Drawing for the job (mm, zero at the part's lowest x, y, z). A direction names the side the tool comes from. Round coordinates to 2 decimals unless told otherwise and drop trailing zeros. Order: outer loops, then holes, each group sorted by start corner. A loop starts at its lowest first (then second) coordinate and runs counter-clockwise, first axis right, second up. Notation, with made-up numbers: (85, 33) - (130, 33) arc R13 ccw to (130, 56) - close; hole circle Ø11 at (59, 50). An arc over 180 degrees is marked (long way). Put each result on its own line as item: value. Start each with the question number.
Item 1: Saw through at D-D on z = 3.65. List the corners of the cut face in (x, y), plus the area to 3 significant figures.
Item 2: Saw through at A-A on z = 2.25. List the corners of the cut face in (x, y), plus the area to 3 significant figures.
Item 3: Mould opens along Y. For the marked faces 3, 4 and 5 say: pulls with the +Y half, pulls with the -Y half, needs draft (parallel to the pull), parting line crosses it, or undercut.
Item 4: Pin check, flat tip, straight feed: pin 1 Ø1.3 at (x, z) = (7.5, 3) entering from +Y. Stop position of the tip, or through.
Item 5: Saw through at C-C on y = 0.45. List the corners of the cut face in (x, z).
Item 6: Probe probe 1 along X at (y, z) = (2.55, 2.2); probe 2 along Y at (x, z) = (10.25, 0.2); probe 3 along Z at (x, y) = (1.5, 3.3). List the from-to ranges inside material, lowest first.
Item 7: Saw through at B-B on x = 1. List the corners of the cut face in (y, z).
Item 8: Which spindle directions (+Z, -Z, +X, -X, +Y, -Y) get a long thin tool onto all of the face, cutting with end or side? Do the marked faces 1 and 2. Say none if no direction does.
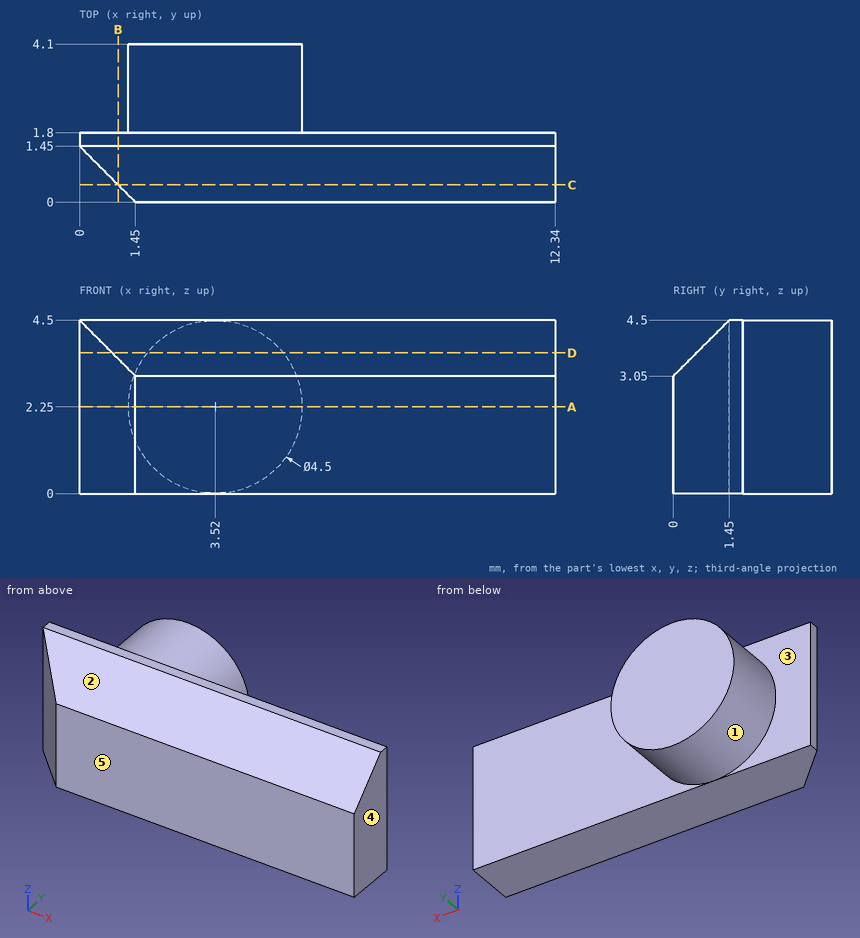
Results found:
1. outline: (0, 1.45) - (0.85, 0.6) - (12.34, 0.6) - (12.34, 1.8) - (5.28, 1.8) - (5.28, 4.1) - (1.76, 4.1) - (1.76, 1.8) - (0, 1.8) - close
1. area: 22.5 mm²
2. outline: (0, 1.45) - (1.45, 0) - (12.34, 0) - (12.34, 1.8) - (5.77, 1.8) - (5.77, 4.1) - (1.27, 4.1) - (1.27, 1.8) - (0, 1.8) - close
2. area: 31.5 mm²
3. face 3: pulls with the +Y half
3. face 4: needs draft
3. face 5: pulls with the -Y half
4. pin 1: stops at y = 1.8
5. outline: (1, 0) - (12.34, 0) - (12.34, 3.5) - (1, 3.5) - close
6. probe 1: x = 1.27 to 5.77
6. probe 2: y = 0 to 1.8
6. probe 3: z = 1.26 to 3.24
7. outline: (0.45, 0) - (1.8, 0) - (1.8, 4.5) - (1.45, 4.5) - (0.45, 3.5) - close
8. face 1: +Y
8. face 2: +Z, +X, -X, -Y
